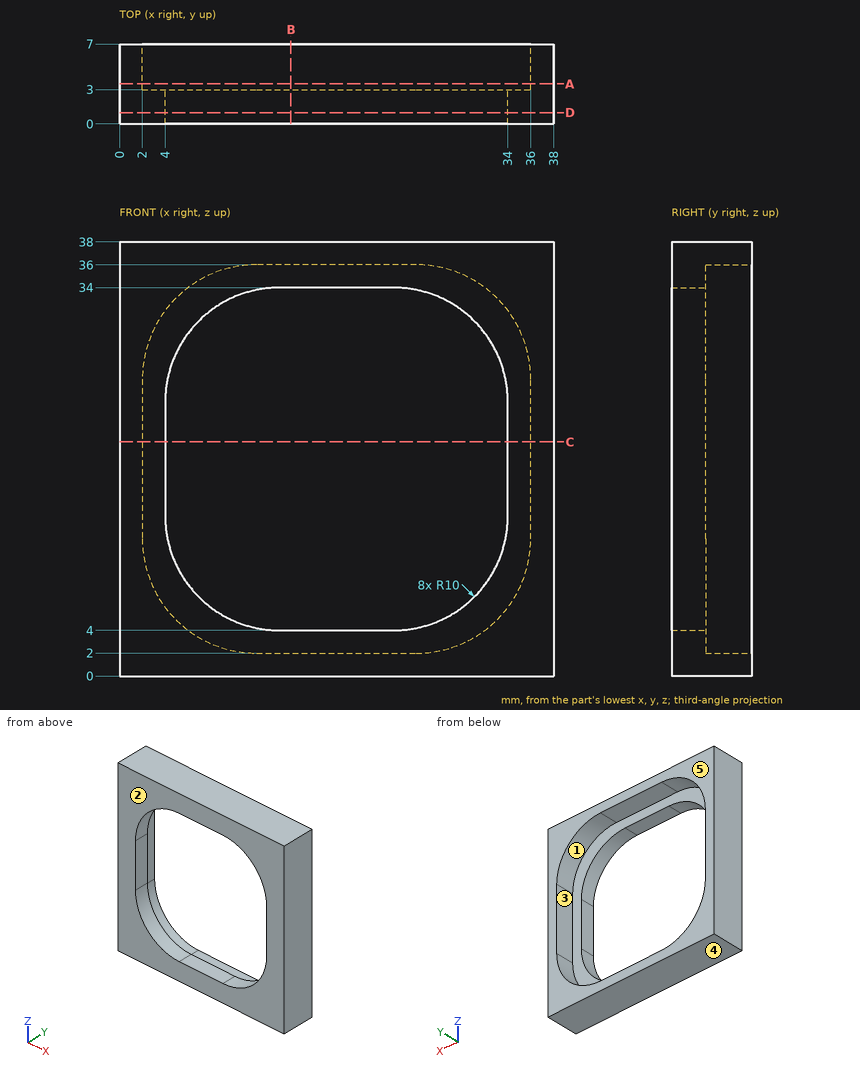
Answer from the drawing. Dimensions are ordinates in mm from the lowest x, y and z of the part. A direction names the side the tool comes from. Round coordinates to 2 decimals unless told otherwise and drop trailing zeros. Write each loop counter-clockwise with the first axis right and the second up, starting at its lowest first coordinate (ties: lowest second). Pieces come first, ordered by that corner, then holes.
1. The part is cut by section D-D, the plane y = 1. Determine the outline of the cut face in (x, z).
2. Given pin 1 Ø12 at (x, z) = (23, 6.5) entering from +Y, flat-ended and moving along its own axis, determine where the tip first touches the part or whether it passes through.
3. The part is cut by section B-B, the plane x = 15. Determine the outline of the cut face in (y, z).
4. The part is cut by section A-A, the plane y = 3.5. Determine the outline of the cut face in (x, z), then the cut area to 3 significant figures.
5. Which of the six approach directions +Z, -Z, +X, -X, +Y, -Y give full straight-line access (tool end or side, diameter ignored) to the marked faces 1 and 2?
6. Determine the mould class of the marked faces 3, 4 and 5 for opening direction Z: pulls with the +Z half, pulls with the -Z half, needs draft (parallel to the pull), parting line crosses it, or undercut.
7. The part is cut by section C-C, the plane z = 20.5. Determine the outline of the cut face in (x, y), then the cut area to 3 significant figures.
8. Straight lines are drawn through the part: L1, parallel to Z at x = 23, y = 6.5; L2, parallel to X at y = 1.5, z = 14.5. For each, find the intervals that lie inside material, in ascending order.
Values:
1. outline: (0, 0) - (38, 0) - (38, 38) - (0, 38) - close; hole (4, 14) arc R10 ccw to (14, 4) - (24, 4) arc R10 ccw to (34, 14) - (34, 24) arc R10 ccw to (24, 34) - (14, 34) arc R10 ccw to (4, 24) - close
2. pin 1: stops at y = 7
3. outline: (0, 0) - (7, 0) - (7, 2) - (3, 2) - (3, 4) - (0, 4) - close; (0, 34) - (3, 34) - (3, 36) - (7, 36) - (7, 38) - (0, 38) - close
4. outline: (0, 0) - (38, 0) - (38, 38) - (0, 38) - close; hole (2, 12) arc R10 ccw to (12, 2) - (26, 2) arc R10 ccw to (36, 12) - (36, 26) arc R10 ccw to (26, 36) - (12, 36) arc R10 ccw to (2, 26) - close
4. area: 374 mm2
5. face 1: +Y
5. face 2: +Z, -Z, +X, -X, -Y
6. face 3: undercut
6. face 4: pulls with the -Z half
6. face 5: needs draft
7. outline: (0, 0) - (4, 0) - (4, 3) - (2, 3) - (2, 7) - (0, 7) - close; (34, 0) - (38, 0) - (38, 7) - (36, 7) - (36, 3) - (34, 3) - close
7. area: 40.0 mm2
8. L1: z = 0 to 2, 36 to 38
8. L2: x = 0 to 4, 34 to 38
